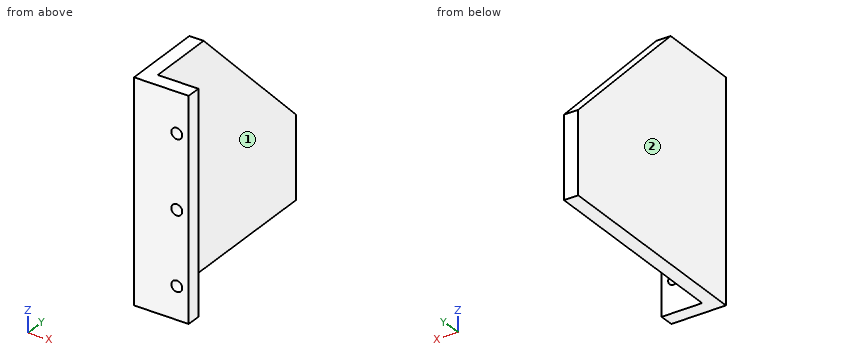
from build123d import *

# Parameters (mm, degrees)
BOSS_EXTRUDE1_DEPTH          = 50.8
F_39_0_0995_DIAMETER_HOLE1_D = 2.5273
CUT_EXTRUDE1_DEPTH           = 3.302


with BuildPart() as part:
    # Sketch4 → Boss-Extrude1 (new body)
    with BuildSketch(Plane.XY):
        Polygon((0, 0), (0, 50.8), (3.302, 50.8), (3.302, 3.302), (12.7, 3.302), (12.7, 0), align=None)
    extrude(amount=BOSS_EXTRUDE1_DEPTH)

    # #39 (0.0995) Diameter Hole1 (through all)
    with Locations(Plane(origin=(0, 0, 0), x_dir=(-1, 0, 0), z_dir=(0, -1, 0))):
        with Locations((-9.929634817, -7.507852782), (-9.929634817, -24.510629703), (-9.929634817, -41.507852782)):
            Hole(F_39_0_0995_DIAMETER_HOLE1_D / 2)

    # Sketch7 → Cut-Extrude1 (cut)
    with BuildSketch(Plane.ZY):
        Polygon((50.8, 50.8), (19.05, 50.8), (50.8, 19.05), align=None)
    extrude(amount=-CUT_EXTRUDE1_DEPTH, mode=Mode.SUBTRACT)


solid = part.part
Model file for the job. Use its own axes, mm. Face numbers are marked on the shaded views. A direction names the side the tool comes from. Give positions to 0.01 mm unless a question says otherwise; leave off trailing zeros. Order: outer loops, then holes, each group sorted by start corner. A loop starts at its lowest first (then second) coordinate and runs counter-clockwise, first axis right, second up. Notation, with made-up numbers: (49.5, -34.75) - (78.5, -34.75) arc R10 ccw to (78.5, -17.75) - close; hole circle Ø3 at (-32, 13.5). An arc over 180 degrees is marked (long way). Return JSON: item names as keys, results as strings.
1) 3-axis set-ups, long thin cutter, end or side, ignore diameter. For the marked faces 1 and 2: which of +Z, -Z, +X, -X, +Y, -Y reach the whole face in a straight line?
Geometry says:
{"face 1": "+Z, -Z, +X, +Y", "face 2": "+Z, -Z, -X, +Y, -Y"}
2) Cut at C-C, the plane y = 23. Give the cut face in (x, z), plus the area to 3 significant figures.
Geometry says:
{"outline": "(0, 0) - (3.3, 0) - (3.3, 46.85) - (0, 46.85) - close", "area": "155 mm²"}
3) Cut at A-A, the plane x = 9.5. Give the cut face in (y, z), plus the area to 3 significant figures.
Geometry says:
{"outline": "(0, 0) - (3.3, 0) - (3.3, 6.32) - (0, 6.32) - close; (0, 8.7) - (3.3, 8.7) - (3.3, 23.32) - (0, 23.32) - close; (0, 25.7) - (3.3, 25.7) - (3.3, 40.32) - (0, 40.32) - close; (0, 42.7) - (3.3, 42.7) - (3.3, 50.8) - (0, 50.8) - close", "area": "144 mm²"}
4) Cut at B-B, the plane x = 2.5. Give the cut face in (y, z).
Geometry says:
{"outline": "(0, 0) - (50.8, 0) - (50.8, 19.05) - (19.05, 50.8) - (0, 50.8) - close"}
5) Flat gauge pins, fed straight in: P1, Ø4, axis at x = 9.93, z = 41.51, coming from the +Y side; P2, Ø4, axis at x = 5.5, y = 13.5, coming from the +Z side; P3, Ø2, axis at y = 19, z = 14.5, coming from the +X side. Where does each tip first touch, or does it go through?
Geometry says:
{"P1": "y = 3.3", "P2": "through", "P3": "x = 3.3"}
6) Cut at D-D, the plane z = 5. Give the cut face in (x, y), plus the area to 3 significant figures.
Geometry says:
{"outline": "(0, 0) - (12.7, 0) - (12.7, 3.3) - (3.3, 3.3) - (3.3, 50.8) - (0, 50.8) - close", "area": "199 mm²"}
7) Probe line 1 (Z direction, x = 9.75, y = 3); line 2 (Y direction, x = 9.75, z = 27). List the from-to ranges inside material, lowest first. Write a range as from..to.
Geometry says:
{"line 1": "0..6.26, 8.76..23.26, 25.76..40.26, 42.76..50.8", "line 2": "0..3.3"}
